Geometry: final body of the model. Coordinates: model frame, mm. A direction names the side the tool comes from. Give positions to 0.01 mm unless a question says otherwise; leave off trailing zeros. Loops run counter-clockwise (first coordinate to the right, second up) from the corner with the lowest first, then second, coordinate; pieces in that order, holes last. Notation, with made-up numbers: (-35.5, 27) - (7.5, 27) arc R9 cw to (7.5, 39) - close; hole circle Ø7 at (61.25, 71.5). An arc over 180 degrees is marked (long way). Use CSV: the item, a comma, the result in double quotes. Start each with the question number.
```python
from build123d import *

# Parameters (mm, degrees)
CUT_EXTRUDE_1_DEPTH      = 185.932420089
CUT_EXTRUDE_1_DEPTH_BACK = 185.932420089
SKETCH_2_W               = 30
SKETCH_2_H               = 10
CUT_EXTRUDE_2_DEPTH      = 185.932420089
CUT_EXTRUDE_2_DEPTH_BACK = 185.932420089
SKETCH_3_R               = 5
SKETCH_3_R_2             = 8
CUT_EXTRUDE_3_DEPTH      = 185.932420219
CUT_EXTRUDE_3_DEPTH_BACK = 185.932420219
SKETCH_5_R               = 5
SKETCH_6_W               = 36
SKETCH_6_H               = 4.5
CUT_EXTRUDE_4_DEPTH      = 6
CHAMFER_1_SIZE           = 1.5
CHAMFER_2_SIZE           = 2.5


with BuildPart() as part:
    # Эскиз1 → Повернуть1 (revolve)
    with BuildSketch(Plane.XY, mode=Mode.PRIVATE) as revolve_1_sk:
        Polygon((0, 13), (0, 20), (60, 20), (60, 30), (110, 30), (110, 21), (180, 21), (180, 13), align=None)
    revolve(revolve_1_sk.sketch.rotate(Axis((0, 0, 0), (1, 0, 0)), 90), axis=Axis((0, 0, 0), (1, 0, 0)))

    # Эскиз2 → Вырез-Вытянуть1 (cut, two sides: drawn at the far end of the back side and taken through both)
    with BuildSketch(Plane.XY.offset(-CUT_EXTRUDE_1_DEPTH_BACK)):
        with Locations((85, 25)):
            Rectangle(SKETCH_2_W, SKETCH_2_H)
    extrude(amount=CUT_EXTRUDE_1_DEPTH + CUT_EXTRUDE_1_DEPTH_BACK, mode=Mode.SUBTRACT)

    # Эскиз3 → Вырез-Вытянуть2 (cut, two sides: drawn at the far end of the back side and taken through both)
    with BuildSketch(Plane(origin=(0, 0, 0), x_dir=(1, 0, 0), z_dir=(0, 1, 0)).offset(-CUT_EXTRUDE_2_DEPTH_BACK)):
        with Locations(Location((30, 0, 0), (0, 0, 270))):
            Circle(SKETCH_3_R)
        with Locations(Location((85, 0, 0), (0, 0, 270))):
            Circle(SKETCH_3_R_2)
    extrude(amount=CUT_EXTRUDE_2_DEPTH + CUT_EXTRUDE_2_DEPTH_BACK, mode=Mode.SUBTRACT)

    # Эскиз5 → Вырез-Вытянуть3 (cut, two sides: drawn at the far end of the back side and taken through both)
    with BuildSketch(Plane.XY.offset(-CUT_EXTRUDE_3_DEPTH_BACK)):
        with Locations((30, 0)):
            Circle(SKETCH_5_R)
    extrude(amount=CUT_EXTRUDE_3_DEPTH + CUT_EXTRUDE_3_DEPTH_BACK, mode=Mode.SUBTRACT)

    # Эскиз6 → Вырез-Вытянуть4 (cut, symmetric)
    with BuildSketch(Plane.XY):
        with Locations((147, 18.75)):
            Rectangle(SKETCH_6_W, SKETCH_6_H)
    extrude(amount=CUT_EXTRUDE_4_DEPTH, both=True, mode=Mode.SUBTRACT)

    # Фаска1
    chamfer_1_edges = [part.edges().sort_by_distance(p)[0] for p in [
        (0, 0, -13),
        (0, 0, -20),
    ]]
    chamfer(chamfer_1_edges, length=CHAMFER_1_SIZE)

    # Фаска2
    chamfer_2_edges = [part.edges().sort_by_distance(p)[0] for p in [
        (180, 0, -13),
        (180, 0, -21),
    ]]
    chamfer(chamfer_2_edges, length=CHAMFER_2_SIZE)


solid = part.part
```
Item 1: Section D-D (y = -25). Output: boundary loops of the cut face in (x, z), plus the area to 3 significant figures.
Item 2: Ray query, probe 1 along X at (y, z) = (18, 0); probe 2 along Y at (x, z) = (67, 0); probe 3 along X at (y, z) = (0, -16). Return the intervals inside material, ascending.
Item 3: Section B-B (x = 158.5). Output: boundary loops of the cut face in (y, z), plus the area to 3 significant figures.
Item 4: Section C-C (x = 85). Output: boundary loops of the cut face in (y, z).
Item 5: Mould query, pull axis Z, two halves, no side actions, for faces 4 (the cylindrical face through (31.16, -6.007, 19.076)), 5 (the cylindrical face through (88.268, -0.572, -12.987)), 6 (the flat face through (165, 19, 0)), 7 (the flat face through (70, 24, 0)). Classes: pulls with the +Z half, pulls with the -Z half, needs draft (parallel to the pull), parting line crosses it, or undercut.
Item 6: Pin query (flat end, axial travel): pin 1 Ø8 at (x, y) = (83, -9) entering from -Z; pin 2 Ø1.1 at (x, y) = (142, 19) entering from +Z; pin 3 Ø2 at (y, z) = (14.5, 20.5) entering from -X. Return the tip coordinate at first contact, or that it passes through.
Item 7: Section A-A (y = 0). Give the number of separate pieces and of enclosed holes in the cut face, plus the area to 3 significant figures.
Item 8: Reachability of faces 1 (the flat face through (110, -20.4, 6.2)), 2 (the flat face through (78, 20, -5)), 3 (the flat face through (129, 19, 0)) from +Z, -Z, +X, -X, +Y, -Y: full face, straight path, thin tool, end or side. Return the list, or none.
Outcome:
1,outline,"(60, -16.58) - (110, -16.58) - (110, 16.58) - (60, 16.58) - close; hole circle Ø16 at (85, 0)"
1,area,"1,460 mm2"
2,probe 1,"x = 0 to 25, 35 to 77, 93 to 129, 165 to 180"
2,probe 2,"y = -30 to -13, 13 to 30"
2,probe 3,"x = 0 to 25, 35 to 180"
3,outline,"(16.5, -6) - (16.5, 6) - (20.12, 6) arc R21 ccw (long way) to (20.12, -6) - close; hole circle Ø26 at (0, 0)"
3,area,"804 mm2"
4,outline,"(-28.91, -8) arc R30 ccw to (20, -22.36) - (20, -8) - (10.25, -8) arc R13 cw to (-10.25, -8) - close; (-28.91, 8) - (-10.25, 8) arc R13 cw to (10.25, 8) - (20, 8) - (20, 22.36) arc R30 ccw to start"
5,face 4,"parting line crosses it"
5,face 5,"undercut"
5,face 6,"undercut"
5,face 7,"needs draft"
6,pin 1,"stops at z = -29.58"
6,pin 2,"stops at z = 10.03"
6,pin 3,"stops at x = 60"
7,separate pieces,"4"
7,enclosed holes,"0"
7,area,"3,500 mm2"
8,face 1,"+X"
8,face 2,"+Z, -Z, +Y"
8,face 3,"+Y"
